The listing builds one solid part. Answer for the finished solid, in the listing's coordinates (mm). Give positions to 0.01 mm unless a question says otherwise; leave off trailing zeros. Order: outer loops, then holes, each group sorted by start corner. A loop starts at its lowest first (then second) coordinate and runs counter-clockwise, first axis right, second up. Notation, with made-up numbers: (76.25, -30) -> (99.25, -30) arc R19 ccw to (99.25, -16) -> close; hole circle Ø7 at (21.25, 42). An arc over 180 degrees is marked (long way). Answer as a JSON object with one key per item and string values. Group by question number.
```python
from build123d import *

# Parameters (mm, degrees)
SKETCH1_W           = 176
SKETCH1_H           = 133.5
SKETCH1_W_2         = 66.5
SKETCH1_H_2         = 10
BOSS_EXTRUDE1_DEPTH = 0.52
SKETCH1_4_W         = 176
SKETCH1_4_H         = 133.5
BOSS_EXTRUDE2_DEPTH = 0.79


with BuildPart() as part:
    # Sketch1 → Boss-Extrude1 (new body, symmetric)
    with BuildSketch(Plane(origin=(0, 0, 0), x_dir=(1, 0, 0), z_dir=(0, 1, 0))):
        Polygon((-93.5, 70.5), (-93.5, -70.5), (93.5, -70.5), (93.5, -5), (93.5, 5), (93.5, 70.5), align=None)
        Rectangle(SKETCH1_W, SKETCH1_H, mode=Mode.SUBTRACT)
        with Locations((126.75, 0)):
            Rectangle(SKETCH1_W_2, SKETCH1_H_2)
        Rectangle(SKETCH1_W, SKETCH1_H)
    extrude(amount=BOSS_EXTRUDE1_DEPTH, both=True)

    # Sketch1_4 → Boss-Extrude2 (add, symmetric)
    with BuildSketch(Plane(origin=(0, 0, 0), x_dir=(1, 0, 0), z_dir=(0, 1, 0))):
        Rectangle(SKETCH1_4_W, SKETCH1_4_H)
    extrude(amount=BOSS_EXTRUDE2_DEPTH, both=True)


solid = part.part
```
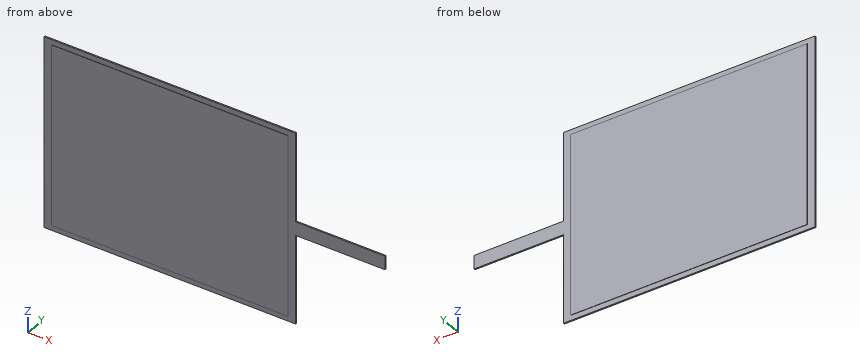
(1) Find the intervals of material crossed by line 1 along Z through (x, y) = (95, -0.2); line 2 along Z through (x, y) = (-53, -0.65); line 3 along X through (y, z) = (0.65, -11), in increasing order. Write a range as [from, to].
(2) A cutting plane is placed at A-A (z = 1.5). Determine the outline of the cut face in (x, y).
(3) A cutting plane is placed at B-B (y = -0.15). Determine the outline of the cut face in (x, z), and give its area (3 significant figures).
(4) Flat-ended cylindrical pins translate along their axes: pin 1 Ø0.8 at (y, z) = (0, -49) entering from +X; pin 2 Ø0.8 at (x, y) = (137.5, -0.5) entering from +Z. Find the tip coordinate at first contact, or state that the pin passes through.
(5) A cutting plane is placed at C-C (x = 27.5). Determine the outline of the cut face in (y, z).
Check sheet entries:
{
 "1": {"line 1": "z = [-5, 5]", "line 2": "z = [-66.75, 66.75]", "line 3": "x = [-88, 88]"},
 "2": {"outline": "(-93.5, -0.52) -> (-88, -0.52) -> (-88, -0.79) -> (88, -0.79) -> (88, -0.52) -> (160, -0.52) -> (160, 0.52) -> (88, 0.52) -> (88, 0.79) -> (-88, 0.79) -> (-88, 0.52) -> (-93.5, 0.52) -> close"},
 "3": {"outline": "(-93.5, -70.5) -> (93.5, -70.5) -> (93.5, -5) -> (160, -5) -> (160, 5) -> (93.5, 5) -> (93.5, 70.5) -> (-93.5, 70.5) -> close", "area": "27,000 mm2"},
 "4": {"pin 1": "stops at x = 93.5", "pin 2": "stops at z = 5"},
 "5": {"outline": "(-0.79, -66.75) -> (-0.52, -66.75) -> (-0.52, -70.5) -> (0.52, -70.5) -> (0.52, -66.75) -> (0.79, -66.75) -> (0.79, 66.75) -> (0.52, 66.75) -> (0.52, 70.5) -> (-0.52, 70.5) -> (-0.52, 66.75) -> (-0.79, 66.75) -> close"}
}
